from build123d import *

# Parameters (mm, degrees)
PAD024_DEPTH    = 18
SKETCH070_R     = 4
POCKET021_DEPTH = 30
SKETCH071_R     = 4
POCKET022_DEPTH = 30
SKETCH074_R     = 4
POCKET025_DEPTH = 18.001


with BuildPart() as part:
    # Sketch066 → Pad024 (new body)
    with BuildSketch(Plane.YZ):
        with BuildLine():
            Line((-600, 750), (-18, 750))
            Line((-18, 375), (-18, 750))
            Line((0, 375), (-18, 375))
            Line((0, 375), (0, 0))
            Line((0, 0), (-300, 0))
            Line((-300, 0), (-300, 375))
            ThreePointArc((-300, 375), (-387.867966, 587.132034), (-600, 675))
            Line((-600, 750), (-600, 675))
        make_face()
    extrude(amount=PAD024_DEPTH)

    # Sketch070 (on Face6 of Pad024) → Pocket021 (cut)
    with BuildSketch(Plane(origin=(0, 0, 750), x_dir=(0, -1, 0), z_dir=(0, 0, 1))):
        with Locations((300, 9)):
            Circle(SKETCH070_R)
        with Locations((450, 9)):
            Circle(SKETCH070_R)
        with Locations((150, 9)):
            Circle(SKETCH070_R)
    extrude(amount=-POCKET021_DEPTH, mode=Mode.SUBTRACT)

    # Sketch071 (on Face6 of Pocket021) → Pocket022 (cut)
    with BuildSketch(Plane.ZX.offset(-18)):
        with Locations((437.5, 9)):
            Circle(SKETCH071_R)
        with Locations((562.5, 9)):
            Circle(SKETCH071_R)
        with Locations((687.5, 9)):
            Circle(SKETCH071_R)
    extrude(amount=-POCKET022_DEPTH, mode=Mode.SUBTRACT)

    # Sketch074 (on Face5 of Pocket022) → Pocket025 (cut, through all)
    with BuildSketch(Plane.YZ.offset(18)):
        with Locations((-225, 384)):
            Circle(SKETCH074_R)
        with Locations((-150, 384)):
            Circle(SKETCH074_R)
        with Locations((-75, 384)):
            Circle(SKETCH074_R)
    extrude(amount=-POCKET025_DEPTH, mode=Mode.SUBTRACT)


with BuildPart() as part_1:
    # Body018001001001010001003001003001001021 placement: moved
    add(part.part.moved(Location((-9, 0, 0))))


solid = part_1.part
Work out the finished part from the listing and answer in its coordinate system (mm). A direction names the side the tool comes from. Round coordinates to 2 decimals unless told otherwise and drop trailing zeros. Order: outer loops, then holes, each group sorted by start corner. A loop starts at its lowest first (then second) coordinate and runs counter-clockwise, first axis right, second up. Notation, with made-up numbers: M -34,43 L 14,43 A21 cw 14,56 Z; hole C -27,56 d11. An arc over 180 degrees is marked long. Put each result on its own line as item: value. Start each with the question number.
Q1. Section C-C, the plane z = 531.5 is taken. Write down the section's boundary in (x, y), and give its area (3 significant figures).
Q2. Flat-ended cylindrical pins translate along their axes: pin 1 (10.5 mm diameter, centred on x = 0, z = 562.5, fed in from +Y); pin 2 (1 mm diameter, centred on x = -6, z = 102.5, fed in from +Y); pin 3 (9 mm diameter, centred on x = 4, y = -12, fed in from +Z); pin 4 (2.5 mm diameter, centred on x = 0.5, y = -151, fed in from +Z). Find the tip coordinate at first contact, or state that the pin passes through.
Q3. Section B-B, the plane z = 67 is taken. Write down the section's boundary in (x, y).
Q4. A tool of negligible diameter and unlimited length cuts with its end or side. For faces 1 (the flat face through (0, 0, 190)), 2 (the flat face through (0, -300, 185)), 3 (the flat face through (-4, -18, 560)), from which of +Z, -Z, +X, -X, +Y, -Y can it reach the whole face along a straight path? Write none if from no direction.
Q5. Section A-A, the plane x = 0 is taken. Give the number of separate pieces and of enclosed holes in the cut face, and give its area (3 significant figures).
Q6. Straight lines are drawn through the part: L1, parallel to Y at x = 3.5, z = 384; L2, parallel to X at y = -150, z = 741; L3, parallel to Y at x = 6, z = 136. For each, find the intervals that lie inside material, in ascending order. Write a range as [from, to].
Findings below:
1. outline: M -9,-344.06 L 9,-344.06 L 9,-18 L -9,-18 Z
1. area: 5,870 mm^2
2. pin 1: stops at y = -18
2. pin 2: stops at y = 0
2. pin 3: stops at z = 375
2. pin 4: stops at z = 720
3. outline: M -9,-300 L 9,-300 L 9,0 L -9,0 Z
4. face 1: +Z, -Z, +X, -X, +Y
4. face 2: -Z, +X, -X, -Y
4. face 3: +Z, +X, -X, +Y
5. separate pieces: 1
5. enclosed holes: 3
5. area: 258,000 mm^2
6. L1: y = [-300.14, -229], [-221, -154], [-146, -79], [-71, -18]
6. L2: x = [-9, -4], [4, 9]
6. L3: y = [-300, 0]
